from build123d import *

# Parameters (mm, degrees)
F0_W           = 50.8
F0_H           = 76.2
F1_DEPTH       = 25.4
F3_D           = 5.6134
F3_CSINK_D     = 10.4394
F3_CSINK_ANGLE = 82
F4_W           = 22.225
F4_H           = 47.625
F5_DEPTH       = 76.201


# Not quite as in the source:
# - a feature names something its author has since deleted; it is built from what else it names


with BuildPart() as f1:
    # F0 (on Right) → F1 (new body)
    with BuildSketch(Plane.YZ):
        Rectangle(F0_W, F0_H)
    extrude(amount=F1_DEPTH)

    # F3 (through all)
    with Locations(Plane.YZ.offset(25.4)):
        with Locations((-3.175, 28.575), (15.875, -28.575)):
            CounterSinkHole(F3_D / 2, F3_CSINK_D / 2, counter_sink_angle=F3_CSINK_ANGLE)

    # F4 (on face) → F5 (cut, through all)
    with BuildSketch(Plane.XY.offset(38.1)):
        with Locations((11.1125, 1.5875)):
            Rectangle(F4_W, F4_H)
    extrude(amount=-F5_DEPTH, mode=Mode.SUBTRACT)


solid = f1.part
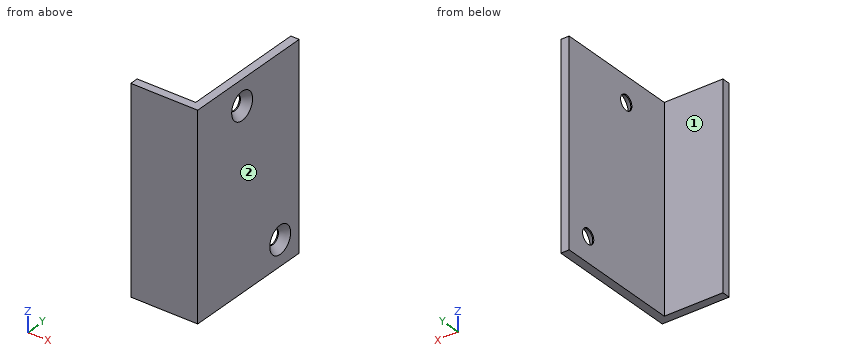
Input: part model. Units: mm. Frame: model coordinates. Face numbers are marked on the shaded views. A direction names the side the tool comes from. Give positions to 0.01 mm unless a question says otherwise; leave off trailing zeros. Loops run counter-clockwise (first coordinate to the right, second up) from the corner with the lowest first, then second, coordinate; pieces in that order, holes last. Notation, with made-up numbers: (-9, -4.75) -> (2, -4.75) arc R8 ccw to (2, 1.25) -> close; hole circle Ø6 at (24, -18.75). An arc over 180 degrees is marked (long way). Answer as a JSON object with one key per item and string values. Group by question number.
Item 1: Pin query (flat end, axial travel): P1, Ø5, axis at x = 19.5, z = 24.5, coming from the +Y side (3 decimals); P2, Ø3, axis at y = 14.5, z = 23, coming from the -X side (3 decimals); P3, Ø1.5, axis at y = -3, z = 29, coming from the -X side; P4, Ø8, axis at x = 21.5, z = 28.5, coming from the +Y side. Return the tip coordinate at first contact, or that it passes through.
Item 2: Line query: probe 1 along X at (y, z) = (8, 0) (3 decimals); probe 2 along Y at (x, z) = (18.25, 18) (3 decimals); probe 3 along X at (y, z) = (13, -32) (3 decimals). Output: solid intervals per line, ascending.
Item 3: Cut plane C-C, the plane x = 12.25. Return the cut outline in (y, z) (3 decimals).
Item 4: Cut plane A-A, the plane z = 6. Return the cut outline in (x, y) (3 decimals), and give its area (3 significant figures).
Item 5: Cut plane B-B, the plane y = 9.5. Return the cut outline in (x, z) (3 decimals).
Item 6: Reachability of the marked faces 1 and 2 from +Z, -Z, +X, -X, +Y, -Y: full face, straight path, thin tool, end or side. Return the list, or none.
Checks:
{
 "1": {"P1": "stops at y = -22.225", "P2": "stops at x = 22.225", "P3": "passes through", "P4": "stops at y = 25.4"},
 "2": {"probe 1": "x = 22.225 to 25.4", "probe 2": "y = -25.4 to -22.225", "probe 3": "x = 22.225 to 24.54"},
 "3": {"outline": "(-25.4, -38.1) -> (-22.225, -38.1) -> (-22.225, 38.1) -> (-25.4, 38.1) -> close"},
 "4": {"outline": "(0, -25.4) -> (25.4, -25.4) -> (25.4, 25.4) -> (22.225, 25.4) -> (22.225, -22.225) -> (0, -22.225) -> close", "area": "232 mm²"},
 "5": {"outline": "(22.225, -38.1) -> (25.4, -38.1) -> (25.4, 38.1) -> (22.225, 38.1) -> close"},
 "6": {"face 1": "+Z, -Z, -X, +Y", "face 2": "+Z, -Z, +X, +Y, -Y"}
}
